Can you work these out from the model? Positions are in its coordinate system, mm. Coordinates: 2 decimals unless noted, no trailing zeros. Order: outer loops, then holes, each group sorted by start corner. A loop starts at its lowest first (then second) coordinate and runs counter-clockwise, first axis right, second up. Notation, with made-up numbers: (85.25, -37) -> (128.25, -37) arc R22 ccw to (128.25, -16) -> close; hole circle Ø9 at (51.5, 82.25). An arc over 180 degrees is marked (long way). Return JSON: item names as keys, results as strings. Group by question number.
1) For pin 1 (1.5 mm diameter, centred on x = 65.5, z = 3, fed in from -Y); pin 2 (1.2 mm diameter, centred on y = 45, z = 2.5, fed in from +X); pin 3 (2 mm diameter, centred on x = 16, z = 2.5, fed in from -Y), each with a flat end and sliding along its axis, tell me the tip position at first contact or that it passes through.
2) If we section it at A-A, the plane z = 2.5: State how many separate pieces and enclosed holes the cut face has, then the cut area to 3 significant figures.
3) If I drill on probe 1 along Y at (x, z) = (68, -0.25); probe 2 along Y at (x, z) = (90, 2.25); probe 3 along Y at (x, z) = (43, 1), over which ranges is the centre line in solid material (lowest first)? Write a range as from..to.
4) If we section it at B-B, the plane x = 4: Please give me the cut outline in (y, z), then the cut area to 3 significant figures.
5) If we section it at D-D, the plane y = 32: Please give me the cut outline in (x, z), then the cut area to 3 significant figures.
6) If we section it at C-C, the plane y = 76: Please give me the cut outline in (x, z).
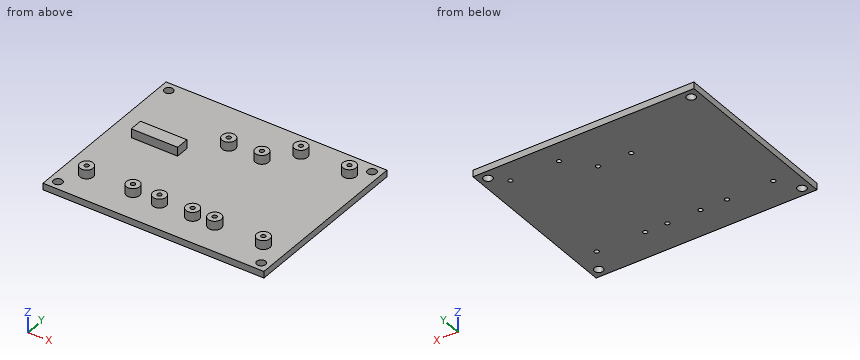
Autodesk Fusion 360 part; units mm, degrees
sketch "mount" plane through (0, 0, 0) normal (0, 0, 1) x (1, 0, 0) in component "Mount"
  line L0 (0, 0) -> (100, 0)
  line L1 (100, 0) -> (100, 80)
  line L2 (100, 80) -> (0, 80)
  line L3 (0, 80) -> (0, 0)
  line L4 (0, 14) -> (100, 14) construction
  circle A0 centre (10, 14) radius 3
  circle A1 centre (31, 14) radius 3
  circle A2 centre (43, 14) radius 3
  circle A3 centre (58, 14) radius 3
  circle A4 centre (68, 14) radius 3
  circle A5 centre (90, 14) radius 3
  line L5 (0, 59) -> (100, 59) construction
  line L6 (0, 70) -> (100, 70) construction
  line L7 (43, 14) -> (43, 59) construction
  line L8 (58, 14) -> (58, 59) construction
  line L9 (68, 14) -> (68, 70) construction
  line L10 (90, 14) -> (90, 70) construction
  circle A6 centre (43, 59) radius 3
  circle A7 centre (58, 59) radius 3
  circle A8 centre (68, 70) radius 3
  circle A9 centre (90, 70) radius 3
  circle A10 centre (4, 76) radius 2
  circle A11 centre (96, 76) radius 2
  line L11 (4, 76) -> (102.7683, 76) construction
  line L12 (96, 76) -> (96, -6.5812) construction
  line L13 (103.6465, 4) -> (-5.3628, 4) construction
  line L14 (4, 83.8921) -> (4, 81.4648) construction
  line L15 (4, 81.4648) -> (4, -6.5812) construction
  circle A12 centre (4, 4) radius 2
  circle A13 centre (96, 4) radius 2
  line L16 (10, 49) -> (31, 49)
  line L17 (31, 49) -> (31, 43)
  line L18 (31, 43) -> (10, 43)
  line L19 (10, 43) -> (10, 49)
  line L20 (10, 14) -> (10, 67.4002) construction
  circle A14 centre (10, 14) radius 1
  circle A15 centre (31, 14) radius 1
  circle A16 centre (43, 14) radius 1
  circle A17 centre (58, 14) radius 1
  circle A18 centre (68, 14) radius 1
  circle A19 centre (90, 14) radius 1
  circle A20 centre (58, 59) radius 1
  circle A21 centre (43, 59) radius 1
  circle A22 centre (68, 70) radius 1
  circle A23 centre (90, 70) radius 1
  dimension "d1" = 100
  dimension "d2" = 80
  dimension "d3" = 14
  dimension "d4" = 6
  dimension "d5" = 6
  dimension "d6" = 6
  dimension "d7" = 6
  dimension "d8" = 6
  dimension "d9" = 6
  dimension "d10" = 10
  dimension "d11" = 22
  dimension "d12" = 10
  dimension "d13" = 15
  dimension "d14" = 10
  dimension "d15" = 21
  dimension "d16" = 45
  dimension "d17" = 56
  dimension "d31" = 6
  dimension "d32" = 6
  dimension "d33" = 6
  dimension "d34" = 6
  dimension "d38" = 4
  dimension "d40" = 4
  dimension "d41" = 4
  dimension "d42" = 4
  dimension "d43" = 4
  dimension "d44" = 4
  dimension "d45" = 4
  dimension "d46" = 4
  dimension "d47" = 21
  dimension "d48" = 6
  dimension "d49" = 29
  dimension "d50" = 2
  dimension "d51" = 2
  dimension "d52" = 2
  dimension "d53" = 2
  dimension "d54" = 2
  dimension "d55" = 2
  dimension "d56" = 2
  dimension "d57" = 2
  dimension "d58" = 2
  dimension "d59" = 2
extrude "Extrude1" add sketch "mount" against normal blind 3 contours L0 L1 L2 L3 | A0 | A1 | A2 | A3 | A4 | A5 | A6 | A7 | A8 | A9 | L16 L17 L18 L19 in component "Mount"
extrude "Extrude2" add sketch "mount" along normal blind 4 and the other way blind 3 contours A0 | A1 | A2 | A3 | A4 | A5 | A6 | A7 | A8 | A9 | L16 L17 L18 L19 in component "Mount"
component "Mount" placed x (1, 0, 0) y (0, 1, 0) z (0, 0, 1) at (0, 0, 0)
Result sheet:
{
 "1": {"pin 1": "stops at y = 11.56", "pin 2": "stops at x = 31", "pin 3": "stops at y = 43"},
 "2": {"separate pieces": "11", "enclosed holes": "10", "area": "377 mm2"},
 "3": {"probe 1": "y = 0..13, 15..69, 71..80", "probe 2": "y = 11..13, 15..17, 67..69, 71..73", "probe 3": "y = 11..13, 15..17, 56..58, 60..62"},
 "4": {"outline": "(0, -3) -> (2, -3) -> (2, 0) -> (0, 0) -> close; (6, -3) -> (74, -3) -> (74, 0) -> (6, 0) -> close; (78, -3) -> (80, -3) -> (80, 0) -> (78, 0) -> close", "area": "216 mm2"},
 "5": {"outline": "(0, -3) -> (100, -3) -> (100, 0) -> (0, 0) -> close", "area": "300 mm2"},
 "6": {"outline": "(0, -3) -> (2, -3) -> (2, 0) -> (0, 0) -> close; (6, -3) -> (94, -3) -> (94, 0) -> (6, 0) -> close; (98, -3) -> (100, -3) -> (100, 0) -> (98, 0) -> close"}
}
